Geometry check sheet. Reference: the model listing, model coordinates, mm. Face numbers are marked on the shaded views. A direction names the side the tool comes from. Give positions to 0.01 mm unless a question says otherwise; leave off trailing zeros. Write each loop counter-clockwise with the first axis right and the second up, starting at its lowest first coordinate (ties: lowest second). Pieces come first, ordered by that corner, then holes. Notation, with made-up numbers: M 74.25,-36 L 108.25,-36 A31 cw 108.25,0 Z; hole C 40.5,-19 d11. An arc over 180 degrees is marked long. One line per item, written item: value. Start each with the question number.
1. Cross-section at B-B on x = 0. Record the cut outline in (y, z) (3 decimals).
2. Release check for a two-part mould opening along Y. For the marked faces 6, 7 and 8 record: pulls with the +Y half, pulls with the -Y half, needs draft (parallel to the pull), parting line crosses it, or undercut.
3. Scan lines: line 1 (Y direction, x = 0, z = 10) (3 decimals); line 2 (Y direction, x = 36, z = 1.25); line 3 (X direction, y = 31, z = 6.75). Record each from-to range of solid material in increasing order.
4. Cross-section at A-A on y = 0. Record the cut outline in (x, z) (3 decimals).
5. Gauge pin test, flat ends, axial feed: pin 1 (5 mm diameter, centred on x = 0, y = 0, fed in from -Z); pin 2 (5 mm diameter, centred on x = -4.5, z = 11.5, fed in from +Y); pin 3 (4 mm diameter, centred on x = -26, z = 2, fed in from -Y); pin 4 (3 mm diameter, centred on y = 5.5, z = 3, fed in from +X). Record the tip position at first contact, or that the pin passes through.
6. Tool access check on the marked faces 1, 2, 3, 4 and 5. Record the directions out of +Z, -Z, +X, -X, +Y, -Y that give a thin tool (end or side, any length) a straight path to the whole face; none if there is none.
from build123d import *

# Parameters (mm, degrees)
SKETCH1_R        = 3.175
EXTRUSION2_DEPTH = 12.7


with BuildPart() as part:
    # Sketch1 → Extrusion2 (new body)
    with BuildSketch(Plane.XY):
        with BuildLine():
            Line((-14.233622753, 38.567186329), (-16.273931786, 37.751596287))
            ThreePointArc((-16.273931786, 37.751596287), (-16.466248372, 34.463305312), (-16.071921005, 31.19308374))
            ThreePointArc((-16.071921005, 31.19308374), (-17.005853093, 30.69390947), (-17.924297324, 30.166781125))
            ThreePointArc((-17.924297324, 30.166781125), (-20.487810109, 32.23517311), (-23.377716537, 33.815769214))
            Line((-23.377716537, 33.815769214), (-25.151096514, 32.51839821))
            ThreePointArc((-25.151096514, 32.51839821), (-24.51960641, 29.285587753), (-23.324396528, 26.216171433))
            ThreePointArc((-23.324396528, 26.216171433), (-24.10484783, 25.500420175), (-24.863345957, 24.761444744))
            ThreePointArc((-24.863345957, 24.761444744), (-27.860709444, 26.127334686), (-31.052902414, 26.939582953))
            Line((-31.052902414, 26.939582953), (-32.447925349, 25.241949579))
            ThreePointArc((-32.447925349, 25.241949579), (-31.0323074, 22.26774901), (-29.111314436, 19.592000659))
            ThreePointArc((-29.111314436, 19.592000659), (-29.689246325, 18.704645697), (-30.240139123, 17.800255724))
            ThreePointArc((-30.240139123, 17.800255724), (-33.483017939, 18.377819734), (-36.776920227, 18.370683619))
            Line((-36.776920227, 18.370683619), (-37.7059317, 16.379456422))
            ThreePointArc((-37.7059317, 16.379456422), (-35.595134387, 13.850745701), (-33.069061394, 11.736792429))
            ThreePointArc((-33.069061394, 11.736792429), (-33.408160285, 10.733589538), (-33.716833132, 9.720611171))
            ThreePointArc((-33.716833132, 9.720611171), (-37.001465276, 9.47355878), (-40.190108886, 8.64748667))
            Line((-40.190108886, 8.64748667), (-40.594735688, 6.487781779))
            ThreePointArc((-40.594735688, 6.487781779), (-37.921388171, 4.563449101), (-34.948957606, 3.144118365))
            ThreePointArc((-34.948957606, 3.144118365), (-35.027916668, 2.088102473), (-35.074974514, 1.030184869))
            ThreePointArc((-35.074974514, 1.030184869), (-38.194974467, -0.025960715), (-41.078005196, -1.619063669))
            Line((-41.078005196, -1.619063669), (-40.932823137, -3.811544054))
            ThreePointArc((-40.932823137, -3.811544054), (-37.864901671, -5.01058579), (-34.632882277, -5.646112218))
            ThreePointArc((-34.632882277, -5.646112218), (-34.446740222, -6.688587749), (-34.22922625, -7.724971737))
            ThreePointArc((-34.22922625, -7.724971737), (-36.988552942, -9.523849001), (-39.384819364, -11.783882284))
            Line((-39.384819364, -11.783882284), (-38.698950767, -13.871376555))
            ThreePointArc((-38.698950767, -13.871376555), (-35.429224142, -14.269787147), (-32.140695585, -14.081576806))
            ThreePointArc((-32.140695585, -14.081576806), (-31.701148402, -15.045009405), (-31.232729815, -15.994739958))
            ThreePointArc((-31.232729815, -15.994739958), (-33.4580046, -18.423318829), (-35.216940485, -21.208276236))
            Line((-35.216940485, -21.208276236), (-34.033480996, -23.059619453))
            ThreePointArc((-34.033480996, -23.059619453), (-30.76739816, -22.632365298), (-27.628990783, -21.632244135))
            ThreePointArc((-27.628990783, -21.632244135), (-26.96365684, -22.456097788), (-26.273766099, -23.259499844))
            ThreePointArc((-26.273766099, -23.259499844), (-27.82516678, -26.165183779), (-28.836251716, -29.300076195))
            Line((-28.836251716, -29.300076195), (-27.229562447, -30.798941653))
            ThreePointArc((-27.229562447, -30.798941653), (-24.172343397, -29.572868701), (-21.381254878, -27.823678007))
            ThreePointArc((-21.381254878, -27.823678007), (-20.531939552, -28.456186959), (-19.663925031, -29.062779812))
            ThreePointArc((-19.663925031, -29.062779812), (-20.443971397, -32.262994003), (-20.643675199, -35.550844607))
            Line((-20.643675199, -35.550844607), (-18.714710347, -36.603053078))
            ThreePointArc((-18.714710347, -36.603053078), (-16.058451399, -34.655200002), (-13.790056095, -32.266847861))
            ThreePointArc((-13.790056095, -32.266847861), (-12.810124992, -32.668269249), (-11.818527235, -33.039938438))
            ThreePointArc((-11.818527235, -33.039938438), (-11.778206103, -36.333601659), (-11.153980648, -39.567822706))
            Line((-11.153980648, -39.567822706), (-9.023944168, -40.107260062))
            ThreePointArc((-9.023944168, -40.107260062), (-6.935547841, -37.560017634), (-5.332377371, -34.682572995))
            ThreePointArc((-5.332377371, -34.682572995), (-4.283403166, -34.827684036), (-3.230527907, -34.941076221))
            ThreePointArc((-3.230527907, -34.941076221), (-2.372372803, -38.121235497), (-0.963440471, -41.098608985))
            Line((-0.963440471, -41.098608985), (1.233829612, -41.091380392))
            ThreePointArc((1.233829612, -41.091380392), (2.623141695, -38.104801222), (3.460354235, -34.919064515))
            ThreePointArc((3.460354235, -34.919064515), (4.512460635, -34.798747349), (5.560457371, -34.64673768))
            ThreePointArc((5.560457371, -34.64673768), (7.182525405, -37.513571908), (9.287636214, -40.04701851))
            Line((9.287636214, -40.04701851), (11.414077338, -39.493578168))
            ThreePointArc((11.414077338, -39.493578168), (12.017009592, -36.255320009), (12.035659057, -32.961462787))
            ThreePointArc((12.035659057, -32.961462787), (13.024789938, -32.583277384), (14.002058661, -32.175417188))
            ThreePointArc((14.002058661, -32.175417188), (16.286119127, -34.548792632), (18.955136559, -36.47912658))
            Line((18.955136559, -36.47912658), (20.877136608, -35.414249181))
            ThreePointArc((20.877136608, -35.414249181), (20.65580458, -32.127783703), (19.854719157, -28.932771129))
            ThreePointArc((19.854719157, -28.932771129), (20.718723787, -28.320480269), (21.563859111, -27.682396902))
            ThreePointArc((21.563859111, -27.682396902), (24.366396088, -29.413185652), (27.431615961, -30.619116966))
            Line((27.431615961, -30.619116966), (29.028408604, -29.109712673))
            ThreePointArc((29.028408604, -29.109712673), (27.9967194, -25.981540589), (26.426234232, -23.086127053))
            ThreePointArc((26.426234232, -23.086127053), (27.110824023, -22.278203223), (27.770722986, -21.44998981))
            ThreePointArc((27.770722986, -21.44998981), (30.915642769, -22.429440044), (34.184466045, -22.835195624))
            Line((34.184466045, -22.835195624), (35.355718928, -20.97610586))
            ThreePointArc((35.355718928, -20.97610586), (33.578497375, -18.202781726), (31.337291821, -15.78889671))
            ThreePointArc((31.337291821, -15.78889671), (31.799451478, -14.836104734), (32.232650202, -13.869800971))
            ThreePointArc((32.232650202, -13.869800971), (35.522345915, -14.036370229), (38.789380407, -13.616454959))
            Line((38.789380407, -13.616454959), (39.461499403, -11.524493171))
            ThreePointArc((39.461499403, -11.524493171), (37.050414867, -9.280275142), (34.279312115, -7.499591919))
            ThreePointArc((34.279312115, -7.499591919), (34.490002447, -6.461799222), (34.669281463, -5.418121527))
            ThreePointArc((34.669281463, -5.418121527), (37.897049426, -4.761343649), (40.95701534, -3.542142351))
            Line((40.95701534, -3.542142351), (41.087768741, -1.348754192))
            ThreePointArc((41.087768741, -1.348754192), (38.194318531, 0.225345259), (35.067437158, 1.260939814))
            ThreePointArc((35.067437158, 1.260939814), (35.013419717, 2.318524899), (34.927514264, 3.373998419))
            ThreePointArc((34.927514264, 3.373998419), (37.890541945, 4.812855662), (40.55117037, 6.754736088))
            Line((40.55117037, 6.754736088), (40.132342459, 8.911731973))
            ThreePointArc((40.132342459, 8.911731973), (36.938332693, 9.716806389), (33.652146155, 9.942242061))
            ThreePointArc((33.652146155, 9.942242061), (33.336815056, 10.953167575), (32.99112289, 11.954117636))
            ThreePointArc((32.99112289, 11.954117636), (35.503232362, 14.084645553), (37.597346229, 16.627189616))
            Line((37.597346229, 16.627189616), (36.655253504, 18.612261243))
            ThreePointArc((36.655253504, 18.612261243), (33.361375562, 18.597724838), (30.122367045, 17.998836674))
            ThreePointArc((30.122367045, 17.998836674), (29.565535701, 18.899582449), (28.981777932, 19.783115677))
            ThreePointArc((28.981777932, 19.783115677), (30.885124119, 22.471445363), (32.281142551, 25.454895671))
            Line((32.281142551, 25.454895671), (30.874980162, 27.143313689))
            ThreePointArc((30.874980162, 27.143313689), (27.68820051, 26.310079837), (24.699888832, 24.924498184))
            ThreePointArc((24.699888832, 24.924498184), (23.936545003, 25.65846705), (23.151401279, 26.369067803))
            ThreePointArc((23.151401279, 26.369067803), (24.326389939, 29.446281617), (24.936595965, 32.683177014))
            Line((24.936595965, 32.683177014), (23.154718267, 33.968851909))
            ThreePointArc((23.154718267, 33.968851909), (20.27527399, 32.369275759), (17.725425763, 30.284061807))
            ThreePointArc((17.725425763, 30.284061807), (16.80353315, 30.805135801), (15.866336939, 31.298154421))
            ThreePointArc((15.866336939, 31.298154421), (16.239139213, 34.570899701), (16.025191344, 37.857854144))
            Line((16.025191344, 37.857854144), (13.979560266, 38.660002235))
            ThreePointArc((13.979560266, 38.660002235), (11.588377438, 36.394591039), (9.637209004, 33.74076645))
            ThreePointArc((9.637209004, 33.74076645), (8.61469351, 34.016204576), (7.584332296, 34.26066289))
            ThreePointArc((7.584332296, 34.26066289), (7.131523647, 37.523301014), (6.106865014, 40.653783068))
            Line((6.106865014, 40.653783068), (3.92601508, 40.922002439))
            ThreePointArc((3.92601508, 40.922002439), (2.173340512, 38.133100314), (0.943450961, 35.077414647))
            ThreePointArc((0.943450961, 35.077414647), (-0.115439006, 35.089910115), (-1.174223838, 35.070447907))
            ThreePointArc((-1.174223838, 35.070447907), (-2.424191777, 38.117975323), (-4.195178104, 40.895285287))
            Line((-4.195178104, 40.895285287), (-6.374216073, 40.612722729))
            ThreePointArc((-6.374216073, 40.612722729), (-7.378255391, 37.475566652), (-7.809587577, 34.210019876))
            ThreePointArc((-7.809587577, 34.210019876), (-8.838318064, 33.958787549), (-9.858999169, 33.676627702))
            ThreePointArc((-9.858999169, 33.676627702), (-11.827586317, 36.317557055), (-14.233622753, 38.567186329))
        make_face()
        Circle(SKETCH1_R, mode=Mode.SUBTRACT)
    extrude(amount=EXTRUSION2_DEPTH)


solid = part.part
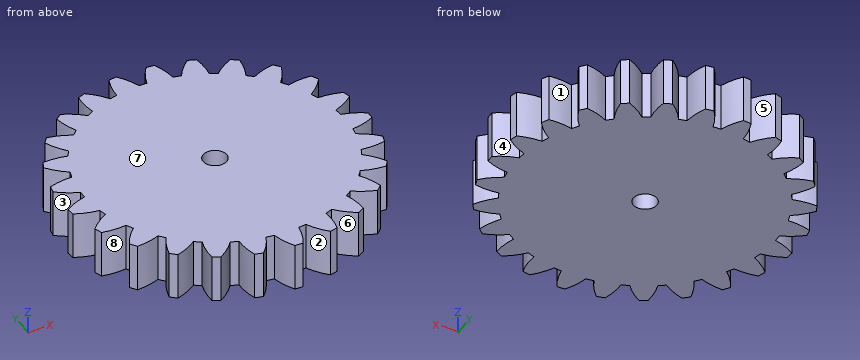
Report:
1. outline: M -41.095,0 L -3.175,0 L -3.175,12.7 L -41.095,12.7 Z; M 3.175,0 L 35.09,0 L 35.09,12.7 L 3.175,12.7 Z
2. face 6: pulls with the -Y half
2. face 7: needs draft
2. face 8: undercut
3. line 1: y = -41.095 to -3.175, 3.175 to 35.09
3. line 2: y = -14.01 to -8.52, -5.22 to 1.02, 3.82 to 9.84, 14.61 to 18.66
3. line 3: x = -24.93 to -18.85, -16.44 to 16.44, 18.5 to 24.69
4. outline: M -38.136,0 L -3.175,0 L -3.175,12.7 L -38.136,12.7 Z; M 3.175,0 L 38.694,0 L 38.694,12.7 L 3.175,12.7 Z
5. pin 1: passes through
5. pin 2: stops at y = 40.9
5. pin 3: stops at y = -30.8
5. pin 4: stops at x = 40.55
6. face 1: +Z, -Z
6. face 2: +Z, -Z, -Y
6. face 3: +Z, -Z, -X
6. face 4: +Z, -Z, +X
6. face 5: +Z, -Z, +Y
